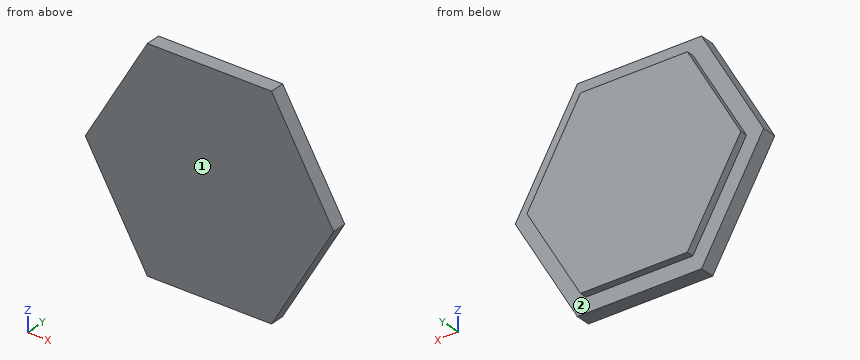
Autodesk Inventor part; units mm, degrees
ref_plane "YZ Plane" through (0, 0, 0) normal (1, 0, 0) x (0, 1, 0)
ref_plane "XZ Plane" through (0, 0, 0) normal (0, 1, 0) x (-1, 0, 0)
ref_plane "XY Plane" through (0, 0, 0) normal (0, 0, 1) x (1, 0, 0)
sketch "Sketch1" plane through (0, 0, 0) normal (0, 1, 0) x (-1, 0, 0)
  line L0 (-107.95, 0) -> (-53.975, 93.4874)
  line L1 (-53.975, 93.4874) -> (53.975, 93.4874)
  line L2 (53.975, 93.4874) -> (107.95, 0)
  line L3 (107.95, 0) -> (53.975, -93.4874)
  line L4 (53.975, -93.4874) -> (-53.975, -93.4874)
  line L5 (-53.975, -93.4874) -> (-107.95, 0)
  line L6 (-95.25, 0.0344) -> (-47.5952, 82.5062)
  line L7 (-47.5952, 82.5062) -> (47.6548, 82.4717)
  line L8 (47.6548, 82.4717) -> (95.25, -0.0344)
  line L9 (95.25, -0.0344) -> (47.5952, -82.5062)
  line L10 (47.5952, -82.5062) -> (-47.6548, -82.4717)
  line L11 (-47.6548, -82.4717) -> (-95.25, 0.0344)
  point P0 (0, 0)
  point P1 (0, 0)
  point P2 (0, 0)
  point P3 (0, 0)
  dimension "d0" = 215.9
  dimension "d1" = 12.7
extrude "Extrusion1" add sketch "Sketch1" along normal blind 12.7 contours L0 L1 L2 L3 L4 L5 | L6 L7 L8 L9 L10 L11
sketch "Sketch2" plane through (0, 12.7, 0) normal (0, 1, 0) x (1, 0, 0)
  line L0 (-107.95, -0.0035) -> (-53.978, 93.4857)
  line L1 (-53.978, 93.4857) -> (53.972, 93.4892)
  line L2 (53.972, 93.4892) -> (107.95, 0.0035)
  line L3 (107.95, 0.0035) -> (53.978, -93.4857)
  line L4 (53.978, -93.4857) -> (-53.972, -93.4892)
  line L5 (-53.972, -93.4892) -> (-107.95, -0.0035)
  line L6 (-92.964, 0.0336) -> (-46.4529, 80.526)
  line L7 (-46.4529, 80.526) -> (46.5111, 80.4924)
  line L8 (46.5111, 80.4924) -> (92.964, -0.0336)
  line L9 (92.964, -0.0336) -> (46.4529, -80.526)
  line L10 (46.4529, -80.526) -> (-46.5111, -80.4924)
  line L11 (-46.5111, -80.4924) -> (-92.964, 0.0336)
  point P0 (0, 0)
  point P1 (0, 0)
  point P2 (0, 0)
  point P3 (0, 0)
  dimension "d4" = 215.9
  dimension "d5" = 14.986
extrude "Extrusion2" add sketch "Sketch2" along normal blind 6.35 contours L6 L7 L8 L9 L10 L11
properties part number "SatelliteBottomFace_v2"
Part model, mm, in its own coordinate system. Face numbers are marked on the shaded views. A direction names the side the tool comes from. Give positions to 0.01 mm unless a question says otherwise; leave off trailing zeros. Order: outer loops, then holes, each group sorted by start corner. A loop starts at its lowest first (then second) coordinate and runs counter-clockwise, first axis right, second up. Notation, with made-up numbers: (-21, 84.25) -> (35, 84.25) arc R16 ccw to (35, 88.25) -> close; hole circle Ø5 at (-28.75, -31). An arc over 180 degrees is marked (long way). Use one line per item in the form item = value.
(1) Flat gauge pins, fed straight in: P1, Ø5, axis at x = 2.5, y = 14.5, coming from the +Z side; P2, Ø1.5, axis at y = 10, z = -38, coming from the +X side; P3, Ø2, axis at x = -79.5, y = 17, coming from the -Z side; P4, Ø3, axis at y = 12, z = -67.5, coming from the -X side. Where does each tip first touch, or does it go through?
Solution:
P1 = 93.49
P2 = 86.44
P3 = -25.07
P4 = -69.84
(2) Drill centre lines: line 1 (Z direction, x = 14, y = 15); line 2 (Y direction, x = -86.5, z = -12); line 3 (X direction, y = 17.25, z = -33.5). Where is each one in solid material? Low to high. Write a range as from..to.
Solution:
line_1 = -80.5..80.51
line_2 = 0..12.7
line_3 = -73.63..73.62
(3) Saw through at D-D (y = 15). Write the cut outline in (x, z).
Solution:
outline = (-92.96, -0.03) -> (-46.45, -80.53) -> (46.51, -80.49) -> (92.96, 0.03) -> (46.45, 80.53) -> (-46.51, 80.49) -> close
(4) Saw through at C-C (z = -38.5). Write the cut outline in (x, y), then the cut area to 3 significant figures.
Solution:
outline = (-85.72, 0) -> (85.72, 0) -> (85.72, 12.7) -> (70.74, 12.7) -> (70.74, 19.05) -> (-70.74, 19.05) -> (-70.74, 12.7) -> (-85.72, 12.7) -> close
area = 3,080 mm²
(5) Saw through at B-B (x = 61.5). Write the cut outline in (y, z), then the cut area to 3 significant figures.
Solution:
outline = (0, -80.45) -> (12.7, -80.45) -> (12.7, -54.51) -> (19.05, -54.51) -> (19.05, 54.49) -> (12.7, 54.49) -> (12.7, 80.45) -> (0, 80.45) -> close
area = 2,740 mm²
(6) Tool access for the marked faces 1 and 2: list every direction of +Z, -Z, +X, -X, +Y, -Y with a clear straight run to the whole face (end or side of a thin tool).
Solution:
face_1 = +Z, -Z, +X, -X, -Y
face_2 = +Y
(7) Saw through at A-A (y = 3.5). Write the cut outline in (x, z) (3 decimals), then the cut area to 3 significant figures.
Solution:
outline = (-107.95, 0) -> (-53.975, -93.487) -> (53.975, -93.487) -> (107.95, 0) -> (53.975, 93.487) -> (-53.975, 93.487) -> close
area = 30,300 mm²
